Here's how the part is built. I have some questions about the finished solid (model axes, mm). Face numbers are marked on the shaded views. A direction names the side the tool comes from. Round coordinates to 2 decimals unless told otherwise and drop trailing zeros. Loops run counter-clockwise (first coordinate to the right, second up) from the corner with the lowest first, then second, coordinate; pieces in that order, holes last. Notation, with made-up numbers: (31, 75.25) - (49, 75.25) arc R16 cw to (49, 94.25) - close; hole circle Ø2 at (-24, 32.25). An arc over 180 degrees is marked (long way). Return JSON: item names as keys, results as strings. Group by question number.
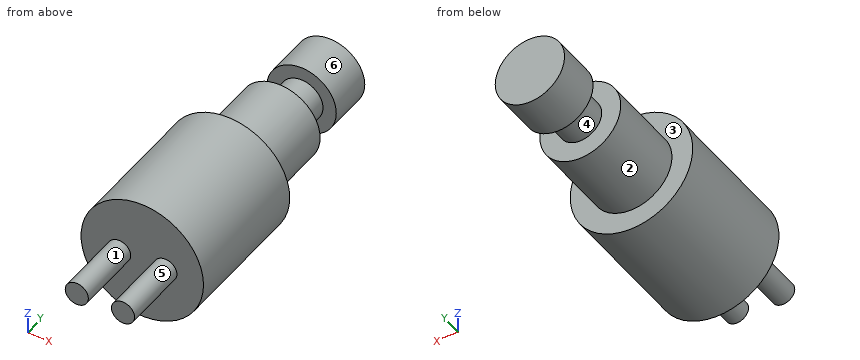
```python
from build123d import *

# Parameters (mm, degrees)
SKETCH2_R           = 5.3
BOSS_EXTRUDE1_DEPTH = 11.8
SKETCH3_R           = 3.5
BOSS_EXTRUDE2_DEPTH = 7
SKETCH4_R           = 1.85
BOSS_EXTRUDE3_DEPTH = 3
SKETCH5_R           = 3
BOSS_EXTRUDE4_DEPTH = 3.9
SKETCH6_R           = 1
BOSS_EXTRUDE5_DEPTH = 5.8


with BuildPart() as part:
    # Sketch2 → Boss-Extrude1 (new body)
    with BuildSketch(Plane(origin=(0, 0, 0), x_dir=(1, 0, 0), z_dir=(0, 1, 0))):
        Circle(SKETCH2_R)
    extrude(amount=BOSS_EXTRUDE1_DEPTH)

    # Sketch3 → Boss-Extrude2 (add)
    with BuildSketch(Plane(origin=(0, 11.8, 0), x_dir=(1, 0, 0), z_dir=(0, 1, 0))):
        Circle(SKETCH3_R)
    extrude(amount=BOSS_EXTRUDE2_DEPTH)

    # Sketch4 → Boss-Extrude3 (add)
    with BuildSketch(Plane(origin=(0, 18.8, 0), x_dir=(1, 0, 0), z_dir=(0, 1, 0))):
        Circle(SKETCH4_R)
    extrude(amount=BOSS_EXTRUDE3_DEPTH)

    # Sketch5 → Boss-Extrude4 (add)
    with BuildSketch(Plane(origin=(0, 21.8, 0), x_dir=(1, 0, 0), z_dir=(0, 1, 0))):
        Circle(SKETCH5_R)
    extrude(amount=BOSS_EXTRUDE4_DEPTH)

    # Sketch6 → Boss-Extrude5 (add)
    with BuildSketch(Plane(origin=(0, 0, 0), x_dir=(-1, 0, 0), z_dir=(0, -1, 0))):
        with Locations((2, 0)):
            Circle(SKETCH6_R)
        with Locations((-2, 0)):
            Circle(SKETCH6_R)
    extrude(amount=BOSS_EXTRUDE5_DEPTH)


solid = part.part
```
Q1. Imagine slicing it at B-B, the plane x = 2.5. List the corners of the cut face in (y, z) for me.
Q2. Please list where these lines run through material, in increasing order: line 1 (Y direction, x = -2, z = 1.5); line 2 (Y direction, x = -4.5, z = 2); line 3 (X direction, y = 17.5, z = 1).
Q3. Imagine slicing it at A-A, the plane z = 0. List the corners of the cut face in (x, y) for me.
Q4. Imagine slicing it at D-D, the plane y = 17. List the corners of the cut face in (x, z) for me.
Q5. Imagine slicing it at C-C, the plane x = 0. List the corners of the cut face in (y, z) for me.
Q6. If we mould it in two halves opening along X, with no side actions, what happens to the marked faces 1, 2 and 3? For each: +X half, -X half, draft (parallel to the pull), parting line (faces both ways), or undercut.
Q7. Will these pins go through, and if not, where does the flat tip stop? pin 1 Ø3 at (x, y) = (-1.5, 20) entering from -Z; pin 2 Ø4 at (y, z) = (20.5, -2) entering from -X; pin 3 Ø1.5 at (y, z) = (19, -2.5) entering from -X; pin 4 Ø3 at (x, z) = (-0.5, 4) entering from +Y.
Q8. For the marked faces 4, 5 and 6, which set-ups out of +Z, -Z, +X, -X, +Y, -Y let a thin tool reach every point of the face, with its end or its side?
Output values:
{
 "1": {"outline": "(-5.8, -0.87) - (0, -0.87) - (0, -4.67) - (11.8, -4.67) - (11.8, -2.45) - (18.8, -2.45) - (18.8, 2.45) - (11.8, 2.45) - (11.8, 4.67) - (0, 4.67) - (0, 0.87) - (-5.8, 0.87) - close; (21.8, -1.66) - (25.7, -1.66) - (25.7, 1.66) - (21.8, 1.66) - close"},
 "2": {"line 1": "y = 0 to 18.8, 21.8 to 25.7", "line 2": "y = 0 to 11.8", "line 3": "x = -3.35 to 3.35"},
 "3": {"outline": "(-5.3, 0) - (-3, 0) - (-3, -5.8) - (-1, -5.8) - (-1, 0) - (1, 0) - (1, -5.8) - (3, -5.8) - (3, 0) - (5.3, 0) - (5.3, 11.8) - (3.5, 11.8) - (3.5, 18.8) - (1.85, 18.8) - (1.85, 21.8) - (3, 21.8) - (3, 25.7) - (-3, 25.7) - (-3, 21.8) - (-1.85, 21.8) - (-1.85, 18.8) - (-3.5, 18.8) - (-3.5, 11.8) - (-5.3, 11.8) - close"},
 "4": {"outline": "circle Ø7 at (0, 0)"},
 "5": {"outline": "(0, -5.3) - (11.8, -5.3) - (11.8, -3.5) - (18.8, -3.5) - (18.8, -1.85) - (21.8, -1.85) - (21.8, -3) - (25.7, -3) - (25.7, 3) - (21.8, 3) - (21.8, 1.85) - (18.8, 1.85) - (18.8, 3.5) - (11.8, 3.5) - (11.8, 5.3) - (0, 5.3) - close"},
 "6": {"face 1": "undercut", "face 2": "parting line", "face 3": "draft"},
 "7": {"pin 1": "stops at z = -3.45", "pin 2": "stops at x = -3.37", "pin 3": "stops at x = -3.02", "pin 4": "stops at y = 25.7"},
 "8": {"face 4": "none", "face 5": "-Y", "face 6": "+Y"}
}
